from build123d import *

# Parameters (mm, degrees)
SKETCH2_W           = 66.5
SKETCH2_H           = 40
BOSS_EXTRUDE1_DEPTH = 5
SKETCH5_W           = 40
SKETCH5_H           = 39
BOSS_EXTRUDE3_DEPTH = 3
SKETCH11_W          = 14.05
SKETCH11_H          = 2.5
SKETCH11_W_2        = 18
SKETCH11_H_2        = 1.5
BOSS_EXTRUDE4_DEPTH = 5.6
FILLET4_R           = 1
SKETCH12_R          = 4
BOSS_EXTRUDE5_DEPTH = 3
FILLET6_R           = 10
SKETCH13_R          = 14
BOSS_EXTRUDE6_DEPTH = 10
SKETCH14_R          = 5
CUT_EXTRUDE1_DEPTH  = 5
SKETCH15_R          = 2.25
CUT_EXTRUDE2_DEPTH  = 3


with BuildPart() as part:
    # Sketch2 → Boss-Extrude1 (new body)
    with BuildSketch(Plane(origin=(0, 0, 0), x_dir=(1, 0, 0), z_dir=(0, 1, 0))):
        Rectangle(SKETCH2_W, SKETCH2_H)
        with BuildLine():
            Line((-27.65, 11.5), (-27.65, -11.5))
            ThreePointArc((-27.65, -11.5), (-26.771320344, -13.621320344), (-24.65, -14.5))
            Line((-24.65, -14.5), (28.85, -14.5))
            ThreePointArc((28.85, -14.5), (30.971320344, -13.621320344), (31.85, -11.5))
            Line((31.85, -11.5), (31.85, 11.5))
            ThreePointArc((31.85, 11.5), (30.971320344, 13.621320344), (28.85, 14.5))
            Line((28.85, 14.5), (-24.65, 14.5))
            ThreePointArc((-24.65, 14.5), (-26.771320344, 13.621320344), (-27.65, 11.5))
        make_face(mode=Mode.SUBTRACT)
    extrude(amount=BOSS_EXTRUDE1_DEPTH)

    # Sketch5 → Boss-Extrude3 (add)
    with BuildSketch(Plane.ZY.offset(33.25)):
        with Locations((0, 19.5)):
            Rectangle(SKETCH5_W, SKETCH5_H)
    extrude(amount=BOSS_EXTRUDE3_DEPTH)

    # Sketch11 → Boss-Extrude4 (add)
    with BuildSketch(Plane(origin=(-33.25, 0, 0), x_dir=(0, 0, -1), z_dir=(1, 0, 0))):
        with Locations((0, 35.75)):
            Rectangle(SKETCH11_W, SKETCH11_H)
        with Locations((0, 7.75)):
            Rectangle(SKETCH11_W_2, SKETCH11_H_2)
    extrude(amount=BOSS_EXTRUDE4_DEPTH)

    # Fillet4
    fillet4_edges = [part.edges().sort_by_distance(p)[0] for p in [
        (-27.65, 7.75, -9),
        (-27.65, 7.75, 9),
    ]]
    fillet(fillet4_edges, radius=FILLET4_R)

    # Sketch12 → Boss-Extrude5 (add)
    with BuildSketch(Plane.ZY.offset(36.25)):
        with Locations((0, 19.5)):
            Circle(SKETCH12_R)
    extrude(amount=BOSS_EXTRUDE5_DEPTH)

    # Fillet6
    fillet6_edges = [part.edges().sort_by_distance(p)[0] for p in [
        (33.25, 2.5, 20),
        (33.25, 2.5, -20),
    ]]
    fillet(fillet6_edges, radius=FILLET6_R)

    # Sketch13 → Boss-Extrude6 (add)
    with BuildSketch(Plane.ZY.offset(39.25)):
        with Locations((0, 19.5)):
            Circle(SKETCH13_R)
    extrude(amount=BOSS_EXTRUDE6_DEPTH)

    # Sketch14 → Cut-Extrude1 (cut)
    with BuildSketch(Plane.ZY.offset(49.25)):
        with Locations((0, 19.5)):
            Circle(SKETCH14_R)
    extrude(amount=-CUT_EXTRUDE1_DEPTH, mode=Mode.SUBTRACT)

    # Sketch15 → Cut-Extrude2 (cut)
    with BuildSketch(Plane.ZY.offset(44.25)):
        with Locations((0, 19.5)):
            Circle(SKETCH15_R)
    extrude(amount=-CUT_EXTRUDE2_DEPTH, mode=Mode.SUBTRACT)


solid = part.part
Could you check a few things on this model? Use its own coordinates, in mm. A direction names the side the tool comes from. Give positions to 0.01 mm unless a question says otherwise; leave off trailing zeros. Order: outer loops, then holes, each group sorted by start corner. A loop starts at its lowest first (then second) coordinate and runs counter-clockwise, first axis right, second up.
1. Will these pins go through, and if not, where does the flat tip stop? P1, Ø4, axis at y = 17, z = 6, coming from the +X side; P2, Ø3.5, axis at y = 19.5, z = 0, coming from the -X side; P3, Ø1.2, axis at x = -31.5, y = 7.5, coming from the -Z side.
2. For faces 5 (the flat face through (-30, 37, 0)), 6 (the flat face through (-31, 8, -9)), 7 (the flat face through (-30, 8.5, 0)), 8 (the cylindrical face through (30.95, 2.46, 13.64)), which set-ups out of +Z, -Z, +X, -X, +Y, -Y let a thin tool reach every point of the face, with its end or its side?
3. Suppose I cut it at D-D (y = 19.5). List the corners of the cut face in (x, z) for me.
4. Suppose I cut it at B-B (x = 16.5). List the corners of the cut face in (y, z) for me.
5. We'd pull the mould along X, two halves only. Please class faces 1 (the cylindrical face through (-26.75, 2.46, -13.64)), 2 (the flat face through (2, 2, 14.5)), 3 (the flat face through (-27.65, 8, 0)), 4 (the cylindrical face through (-42.771, 17.304, -0.488)): pulls with the +X half, pulls with the -X half, needs draft (parallel to the pull), parting line crosses it, or undercut.
6. Suppose I cut it at C-C (y = 4). List the corners of the cut face in (x, z) for me, plus the area to 3 significant figures.
7. I need wall thicknesses on L1, parallel to Y at x = -33, z = -8; L2, parallel to X at y = 2.5, z = 5; L3, parallel to X at y = 9, z = 7. Which ranges of each line are inside material? Lowest first, please.
Solved:
1. P1: stops at x = -33.25
1. P2: stops at x = -41.25
1. P3: stops at z = -9
2. face 5: +Z, -Z, +X, +Y
2. face 6: -Z, +X, +Y
2. face 7: +Z, -Z, +X
2. face 8: +Y, -Y
3. outline: (-49.25, -14) - (-39.25, -14) - (-39.25, -4) - (-36.25, -4) - (-36.25, -20) - (-33.25, -20) - (-33.25, 20) - (-36.25, 20) - (-36.25, 4) - (-39.25, 4) - (-39.25, 14) - (-49.25, 14) - (-49.25, 5) - (-44.25, 5) - (-44.25, 2.25) - (-41.25, 2.25) - (-41.25, -2.25) - (-44.25, -2.25) - (-44.25, -5) - (-49.25, -5) - close
4. outline: (0, -20) - (5, -20) - (5, -14.5) - (0, -14.5) - close; (0, 14.5) - (5, 14.5) - (5, 20) - (0, 20) - close
5. face 1: undercut
5. face 2: undercut
5. face 3: pulls with the +X half
5. face 4: needs draft
6. outline: (-36.25, -20) - (23.25, -20) arc R10 ccw to (33.25, -10) - (33.25, 10) arc R10 ccw to (23.25, 20) - (-36.25, 20) - close; hole (-27.65, -11.5) arc R3 ccw to (-24.65, -14.5) - (28.85, -14.5) arc R3 ccw to (31.85, -11.5) - (31.85, 11.5) arc R3 ccw to (28.85, 14.5) - (-24.65, 14.5) arc R3 ccw to (-27.65, 11.5) - close
6. area: 1,020 mm2
7. L1: y = 0 to 5, 7 to 8.5
7. L2: x = -36.25 to -27.65, 31.85 to 33.25
7. L3: x = -49.25 to -39.25, -36.25 to -33.25
